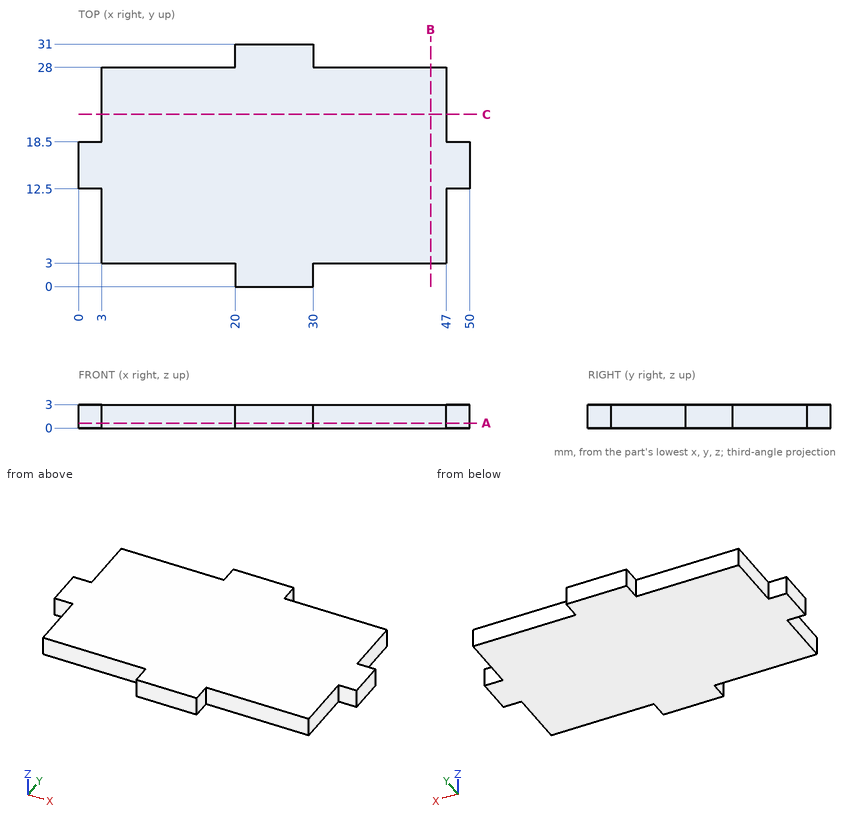
Geometry check sheet. Reference: drawing and pictorial views, mm from the part's lowest x, y, z. Round coordinates to 2 decimals unless told otherwise and drop trailing zeros. Order: outer loops, then holes, each group sorted by start corner. A loop starts at its lowest first (then second) coordinate and runs counter-clockwise, first axis right, second up. Notation, with made-up numbers: (-25, -6) - (9, -6) arc R25 ccw to (9, 27) - close; hole circle Ø9 at (51, 63). An arc over 180 degrees is marked (long way). Use a Markdown table: item, result. Add a question column.
1) Thickness scan on line 1 along X through (y, z) = (9, 0.15); line 2 along Y through (x, z) = (12.5, 2.7); line 3 along Y through (x, z) = (2, 1.8). Record the ranges inside material, lowest first.
2) Gauge pin test, flat ends, axial feed: P1, Ø1.5, axis at y = 30, z = 1, coming from the -X side; P2, Ø1.5, axis at x = 2, z = 2, coming from the -Y side; P3, Ø1, axis at x = 36, z = 0.5, coming from the -Y side. Record the tip position at first contact, or that the pin passes through.
3) Section check B-B (x = 45). Record the cut outline in (y, z).
4) Section check C-C (y = 22). Record the cut outline in (x, z).
5) Section check A-A (z = 0.65). Record the cut outline in (x, y).
Established:
| question | item | result |
|---|---|---|
| 1 | line 1 | 3 to 47 |
| 1 | line 2 | 3 to 28 |
| 1 | line 3 | 12.5 to 18.5 |
| 2 | P1 | x = 20 |
| 2 | P2 | y = 12.5 |
| 2 | P3 | y = 3 |
| 3 | outline | (3, 0) - (28, 0) - (28, 3) - (3, 3) - close |
| 4 | outline | (3, 0) - (47, 0) - (47, 3) - (3, 3) - close |
| 5 | outline | (0, 12.5) - (3, 12.5) - (3, 3) - (20, 3) - (20, 0) - (30, 0) - (30, 3) - (47, 3) - (47, 12.5) - (50, 12.5) - (50, 18.5) - (47, 18.5) - (47, 28) - (30, 28) - (30, 31) - (20, 31) - (20, 28) - (3, 28) - (3, 18.5) - (0, 18.5) - close |
